```python
from build123d import *

# Parameters (mm, degrees)
SKETCH_1_R          = 3.5
SKETCH_1_R_2        = 18
SKETCH_1_R_3        = 5
EXTRUDE_1_DEPTH     = 5.5
SKETCH_2_R          = 17
SKETCH_2_R_2        = 5
EXTRUDE_2_DEPTH     = 6
SKETCH_3_R          = 7
SKETCH_3_R_2        = 5
EXTRUDE_3_DEPTH     = 4
CUT_EXTRUDE_START   = -1
SKETCH_4_R          = 14.65
SKETCH_4_R_2        = 7
CUT_EXTRUDE_1_DEPTH = 1


with BuildPart() as part:
    # 草图1 → 凸台-拉伸1 (new body)
    # profile 1 of 3: a face of its own
    with BuildSketch(Plane(origin=(0, 0, 0), x_dir=(1, 0, 0), z_dir=(0, 1, 0))):
        with BuildLine():
            Line((-14.5934987, 10.537067699), (-30, 4.60495562))
            Line((-30, 4.60495562), (-30, -4.60495562))
            Line((-30, -4.60495562), (-14.5934987, -10.537067699))
            ThreePointArc((-14.5934987, -10.537067699), (-18, 0), (-14.5934987, 10.537067699))
        make_face()
        with Locations(Location((-22.5, 0, 0), (0, 0, 270))):
            Circle(SKETCH_1_R, mode=Mode.SUBTRACT)
    # profile 2 of 3: a face of its own
    with BuildSketch(Plane(origin=(0, 0, 0), x_dir=(1, 0, 0), z_dir=(0, 1, 0))):
        Circle(SKETCH_1_R_2)
        with Locations(Location((0, 0, 0), (0, 0, 270))):
            Circle(SKETCH_1_R_3, mode=Mode.SUBTRACT)
    # profile 3 of 3: a face of its own
    with BuildSketch(Plane(origin=(0, 0, 0), x_dir=(1, 0, 0), z_dir=(0, 1, 0))):
        with BuildLine():
            Line((30, 4.60495562), (14.5934987, 10.537067699))
            ThreePointArc((14.5934987, 10.537067699), (17.127214844, 5.537012886), (18, 0))
            ThreePointArc((18, 0), (17.127214844, -5.537012886), (14.5934987, -10.537067699))
            Line((14.5934987, -10.537067699), (30, -4.60495562))
            Line((30, -4.60495562), (30, 4.60495562))
        make_face()
        with Locations(Location((22.5, 0, 0), (0, 0, 270))):
            Circle(SKETCH_1_R, mode=Mode.SUBTRACT)
    extrude(amount=EXTRUDE_1_DEPTH)

    # 草图2 → 凸台-拉伸2 (add)
    with BuildSketch(Plane(origin=(0, 5.5, 0), x_dir=(1, 0, 0), z_dir=(0, 1, 0))):
        with Locations(Location((0, 0, 0), (0, 0, 270))):
            Circle(SKETCH_2_R)
        with Locations(Location((0, 0, 0), (0, 0, 270))):
            Circle(SKETCH_2_R_2, mode=Mode.SUBTRACT)
    extrude(amount=EXTRUDE_2_DEPTH)

    # 草图3 → 凸台-拉伸3 (add)
    with BuildSketch(Plane(origin=(0, 11.5, 0), x_dir=(1, 0, 0), z_dir=(0, 1, 0))):
        with Locations(Location((0, 0, 0), (0, 0, 270))):
            Circle(SKETCH_3_R)
        with Locations(Location((0, 0, 0), (0, 0, 270))):
            Circle(SKETCH_3_R_2, mode=Mode.SUBTRACT)
    extrude(amount=EXTRUDE_3_DEPTH)

    # 草图4 → 切除-拉伸1 (cut)
    with BuildSketch(Plane(origin=(0, 11.5, 0), x_dir=(1, 0, 0), z_dir=(0, 1, 0)).offset(CUT_EXTRUDE_START)):
        with Locations(Location((0, 0, 0), (0, 0, 270))):
            Circle(SKETCH_4_R)
        with Locations(Location((0, 0, 0), (0, 0, 270))):
            Circle(SKETCH_4_R_2, mode=Mode.SUBTRACT)
    extrude(amount=CUT_EXTRUDE_1_DEPTH, mode=Mode.SUBTRACT)


solid = part.part
```
CAD build for the part. Positions are in the model's coordinates, mm. A direction names the side the tool comes from. Round coordinates to 2 decimals unless told otherwise and drop trailing zeros. Loops run counter-clockwise (first coordinate to the right, second up) from the corner with the lowest first, then second, coordinate; pieces in that order, holes last. Notation, with made-up numbers: M 55.5,68 L 83.5,68 A31 cw 83.5,101 Z; hole C 69.25,31.25 d9. An arc over 180 degrees is marked long. Use a Markdown table: item, result. Add a question column.
(1) Which spindle directions (+Z, -Z, +X, -X, +Y, -Y) get a long thin tool onto all of the face, cutting with end or side? Do faces 1 (the face through (0, 3, -18)), 2 (the face through (3.5, 10.5, 6.3)). Say none if no direction does.
(2) Cut at C-C (y = 3). Give the cut face in (x, z), and give its area (3 significant figures).
(3) Pull direction Z, two halves, no side cores. Call faces 3 (the face through (-6.834, 12.965, -1.517)), 4 (the face through (0, 3, 18)), 5 (the face through (14, 11.5, 5)): +Z half, -Z half, draft (parallel to the pull), parting line (faces both ways), or undercut.
(4) Cut at B-B (z = 0). Give the cut face in (x, y).
(5) Cut at D-D (y = 9). Give the cut face in (x, z).
(6) Cut at A-A (x = 0). Give the cut face in (y, z).
(7) Flat gauge pins, fed straight in: pin 1 (17.5 mm diameter, centred on x = 0, z = 0, fed in from +Y); pin 2 (3 mm diameter, centred on x = -18.5, y = 4, fed in from +Z); pin 3 (8 mm diameter, centred on x = -6.5, y = 11.5, fed in from +Z); pin 4 (12 mm diameter, centred on x = -2, z = 14.5, fed in from +Y). Where does each tip first touch, or does it go through?
(8) Drill centre lines: line 1 (X direction, y = 1.4, z = 0); line 2 (X direction, y = 2.5, z = 1.5); line 3 (Z direction, x = 5.5, y = 11). Where is each one in solid material? Low to high.
Geometry says:
| question | item | result |
|---|---|---|
| 1 | face 1 | -Z, +Y, -Y |
| 1 | face 2 | +Y |
| 2 | outline | M -30,-4.6 L -14.59,-10.54 A18 ccw 14.59,-10.54 L 30,-4.6 L 30,4.6 L 14.59,10.54 A18 ccw -14.59,10.54 L -30,4.6 Z; hole C -22.5,0 d7; hole C 0,0 d10; hole C 22.5,0 d7 |
| 2 | area | 1,230 mm² |
| 3 | face 3 | undercut |
| 3 | face 4 | +Z half |
| 3 | face 5 | draft |
| 4 | outline | M -30,0 L -26,0 L -26,5.5 L -30,5.5 Z; M -19,0 L -5,0 L -5,15.5 L -7,15.5 L -7,10.5 L -14.65,10.5 L -14.65,11.5 L -17,11.5 L -17,5.5 L -19,5.5 Z; M 5,0 L 19,0 L 19,5.5 L 17,5.5 L 17,11.5 L 14.65,11.5 L 14.65,10.5 L 7,10.5 L 7,15.5 L 5,15.5 Z; M 26,0 L 30,0 L 30,5.5 L 26,5.5 Z |
| 5 | outline | C 0,0 d34; hole C 0,0 d10 |
| 6 | outline | M 0,-18 L 5.5,-18 L 5.5,-17 L 11.5,-17 L 11.5,-14.65 L 10.5,-14.65 L 10.5,-7 L 15.5,-7 L 15.5,-5 L 0,-5 Z; M 0,5 L 15.5,5 L 15.5,7 L 10.5,7 L 10.5,14.65 L 11.5,14.65 L 11.5,17 L 5.5,17 L 5.5,18 L 0,18 Z |
| 7 | pin 1 | stops at y = 15.5 |
| 7 | pin 2 | stops at z = 9.61 |
| 7 | pin 3 | stops at z = 16.82 |
| 7 | pin 4 | stops at y = 11.5 |
| 8 | line 1 | x = -30 to -26, -19 to -5, 5 to 19, 26 to 30 |
| 8 | line 2 | x = -30 to -25.66, -19.34 to -4.77, 4.77 to 19.34, 25.66 to 30 |
| 8 | line 3 | z = -16.09 to -13.58, -4.33 to 4.33, 13.58 to 16.09 |
